Check sheet for the modelled part. Datum: model origin and axes. Units: mm. A direction names the side the tool comes from. Give positions to 0.01 mm unless a question says otherwise; leave off trailing zeros. Loops run counter-clockwise (first coordinate to the right, second up) from the corner with the lowest first, then second, coordinate; pieces in that order, holes last. Notation, with made-up numbers: (60, 72.25) -> (95, 72.25) arc R19 ccw to (95, 90.25) -> close; hole circle Ø6 at (-6, 22.5). An arc over 180 degrees is marked (long way). Write each question's results on one line, items separated by ' | '. Start each with the question number.
1. Tool access check on faces 1 (the face through (0.57, 14.4, 3.04)), 2 (the face through (66, 0, 3)), 3 (the face through (4, 0, 3)). Record the directions out of +Z, -Z, +X, -X, +Y, -Y that give a thin tool (end or side, any length) a straight path to the whole face; none if there is none.
2. Cross-section at A-A on z = 4.3. Record the boundary of the cut face in (x, y), and give its area (3 significant figures).
3. Cross-section at B-B on y = -1.5. Record the boundary of the cut face in (x, z).
4. Gauge pin test, flat ends, axial feed: pin 1 Ø1.5 at (y, z) = (-2, 2.5) entering from -X; pin 2 Ø0.9 at (y, z) = (-2, 3.5) entering from +X. Record the tip position at first contact, or that the pin passes through.
5. Material ranges on L1, parallel to Y at x = 66.5, z = 4.7; L2, parallel to X at y = -2, z = 3.3; L3, parallel to X at y = 0.5, z = 1.45, recorded low to high. Write a range as from..to.
from build123d import *

# Parameters (mm, degrees)
SKETCH_1_W      = 70
SKETCH_1_H      = 15
EXTRUDE_1_DEPTH = 6
FILLET_1_R      = 2
SKETCH_2_W      = 58
SKETCH_2_H      = 6
EXTRUDE_2_DEPTH = 3


with BuildPart() as part:
    # Эскиз1 → Бобышка-Вытянуть1 (new body)
    with BuildSketch(Plane.XY):
        with Locations((35, 7.5)):
            Rectangle(SKETCH_1_W, SKETCH_1_H)
    extrude(amount=EXTRUDE_1_DEPTH)

    # Скругление1
    fillet_1_edges = [part.edges().sort_by_distance(p)[0] for p in [
        (0, 15, 3),
        (70, 15, 3),
        (70, 0, 3),
        (0, 0, 3),
    ]]
    fillet(fillet_1_edges, radius=FILLET_1_R)

    # Эскиз2 → Бобышка-Вытянуть2 (add)
    with BuildSketch(Plane.XZ):
        with Locations((35, 3)):
            Rectangle(SKETCH_2_W, SKETCH_2_H)
    extrude(amount=EXTRUDE_2_DEPTH)


solid = part.part
Geometry says:
1) face 1: +Z, -Z, -X, +Y | face 2: +Z, -Z, +X, -Y | face 3: +Z, -Z, -X, -Y
2) outline: (0, 2) arc R2 ccw to (2, 0) -> (6, 0) -> (6, -3) -> (64, -3) -> (64, 0) -> (68, 0) arc R2 ccw to (70, 2) -> (70, 13) arc R2 ccw to (68, 15) -> (2, 15) arc R2 ccw to (0, 13) -> close | area: 1,220 mm^2
3) outline: (6, 0) -> (64, 0) -> (64, 6) -> (6, 6) -> close
4) pin 1: x = 6 | pin 2: x = 64
5) L1: 0..15 | L2: 6..64 | L3: 0.68..69.32
